from build123d import *

# Parameters (mm, degrees)
SKETCH2_R           = 0.9
RESISTOR_BODY_DEPTH = 4.1
LEAD1_PROFILE_R     = 0.25
LEAD2_START         = -7.4
SKETCH6_R           = 0.25
LEAD2_DEPTH         = 7.4


with BuildPart() as part:
    # Sketch2 → Resistor Body (new body)
    with BuildSketch(Plane.XY):
        Circle(SKETCH2_R)
    extrude(amount=RESISTOR_BODY_DEPTH)

    # Lead1: sweep along a path in Lead1 Path
    with BuildLine(Plane(origin=(0, 0, 0), x_dir=(1, 0, 0), z_dir=(0, 1, 0))) as lead1_path:
        Line((5, 7.4), (5, -6.1))
        ThreePointArc((5, -6.1), (4.414213562, -7.514213562), (3, -8.1))
        Line((3, -8.1), (2, -8.1))
        ThreePointArc((2, -8.1), (0.585786438, -7.514213562), (0, -6.1))
        Line((0, -6.1), (0, -4.1))
    # Lead1 Profile → Lead1 (sweep)
    with BuildSketch(Plane(origin=(0, 0, 4.1), x_dir=(-1, 0, 0), z_dir=(0, 0, 1))):
        Circle(LEAD1_PROFILE_R)
    sweep(path=lead1_path.line)

    # Sketch6 → Lead2 (add)
    with BuildSketch(Plane.XY.offset(LEAD2_START)):
        Circle(SKETCH6_R)
    extrude(amount=LEAD2_DEPTH)


solid = part.part
The model under review builds one solid part; all positions refer to its coordinate system, in mm. Give positions to 0.01 mm unless a question says otherwise; leave off trailing zeros. Order: outer loops, then holes, each group sorted by start corner. A loop starts at its lowest first (then second) coordinate and runs counter-clockwise, first axis right, second up. Notation, with made-up numbers: M 58.25,75 L 115.25,75 A30 ccw 115.25,100 Z; hole C 19.5,-0.75 d8. An arc over 180 degrees is marked long. One line per question, with ' | ' between items. Start each with the question number.
1) Consider section A-A, the plane y = 0. Give the boundary of the cut face in (x, z).
2) Mouldability with a two-part tool opening along Z and no side actions: class faces 1 (the face through (0, -0.4, 4.1)), 2 (the face through (0.86, 0.27, 2.02)), 3 (the face through (0, -0.4, 0)) as pulls with the +Z half, pulls with the -Z half, needs draft (parallel to the pull), parting line crosses it, or undercut.
3) Clearance check with flat-ended pins moving along their axes: P1, Ø1.5, axis at x = 1, z = 0, coming from the -Y side; P2, Ø3, axis at x = 2.5, z = 3, coming from the -Y side; P3, Ø1, axis at x = 1, y = -0.5, coming from the -Z side. State where each tip first meets the part, or that it passes through.
4) Consider section B-B, the plane z = -5.75. Give the boundary of the cut face in (x, y).
5) Wall thickness on L1, parallel to Y at x = 5, z = 3; L2, parallel to Z at x = -0.5, y = 0.6; L3, parallel to Z at x = 2.25, y = 0: over which ranges is each line inside the solid? List them lowest first. Write a range as from..to.
6) Consider section C-C, the plane x = 2.5. Give the boundary of the cut face in (y, z), then the cut area to 3 significant figures.
Found:
1) outline: M -0.9,0 L -0.25,0 L -0.25,-7.4 L 0.25,-7.4 L 0.25,0 L 0.9,0 L 0.9,4.1 L 0.25,4.1 L 0.25,6.1 A1.75 cw 2,7.85 L 3,7.85 A1.75 cw 4.75,6.1 L 4.75,-7.4 L 5.25,-7.4 L 5.25,6.1 A2.25 ccw 3,8.35 L 2,8.35 A2.25 ccw -0.25,6.1 L -0.25,4.1 L -0.9,4.1 Z
2) face 1: undercut | face 2: needs draft | face 3: pulls with the -Z half
3) P1: stops at y = -0.86 | P2: passes through | P3: stops at z = 0
4) outline: C 0,0 d0.5; C 5,0 d0.5
5) L1: y = -0.25..0.25 | L2: z = 0..4.1 | L3: z = 7.85..8.35
6) outline: C 0,8.1 d0.5 | area: 0.196 mm²
